from build123d import *

# Parameters (mm, degrees)
SKETCH3_R          = 3.175
CUT_EXTRUDE1_DEPTH = 0.91186
CIRPATTERN1_COUNT  = 8


with BuildPart() as part:
    # Sketch1 → Revolve1 (revolve)
    with BuildSketch(Plane.XY):
        Polygon((-1101.212903226, 25.4), (-1060.572903226, 76.2), (-1040.252903226, 76.2), (-1039.341043226, 76.2), (-1039.341043226, 89.81186), (-1040.252903226, 89.81186), (-1040.252903226, 77.11186), (-1061.011165799, 77.11186), (-1101.924946258, 25.969634426), align=None)
    revolve(axis=Axis((0, 0, 0), (-1, 0, 0)))

    # Sketch3 → Cut-Extrude1 (cut)
    with BuildSketch(Plane.ZY.offset(1040.252903226)):
        with Locations((0, 85.09)):
            Circle(SKETCH3_R)
    cut_extrude1 = extrude(amount=-CUT_EXTRUDE1_DEPTH, mode=Mode.SUBTRACT)

    # CirPattern1: Cut-Extrude1 ×8 about axis
    cirpattern1_axis = Axis((0, 0, 0), (1, 0, 0))
    for i in range(1, CIRPATTERN1_COUNT):
        add(cut_extrude1.rotate(cirpattern1_axis, i * 360 / CIRPATTERN1_COUNT), mode=Mode.SUBTRACT)


solid = part.part
Check sheet for the modelled part. Datum: model origin and axes. Units: mm. A direction names the side the tool comes from. Round coordinates to 2 decimals unless told otherwise and drop trailing zeros. Order: outer loops, then holes, each group sorted by start corner. A loop starts at its lowest first (then second) coordinate and runs counter-clockwise, first axis right, second up. Notation, with made-up numbers: M 38,-10 L 82,-10 A26 ccw 82,20 Z; hole C 16.25,16 d5. An arc over 180 degrees is marked long. One line per item, written item: value. Start each with the question number.
1. Access from +Z, -Z, +X, -X, +Y, -Y to the whole of each face (thin tool, end or side, straight path). Record for faces 4 (the cylindrical face through (-1049.808, -60.47, 46.367)), 5 (the cylindrical face through (-1039.8, 60.03, -63.34)), 6 (the flat face through (-1040.253, 0, 79)).
2. Section check D-D on x = -1051. Enter the section's corners in (y, z), and give its area (3 significant figures).
3. Section check A-A on z = 0. Enter the section's corners in (x, y) (3 decimals), and give its area (3 significant figures).
4. Scan lines: line 1 along Z through (x, y) = (-1039.7, 0) (3 decimals); line 2 along Y through (x, z) = (-1045, 0); line 3 along Z through (x, y) = (-1063, 34.5). Record each from-to range of solid material in increasing order.
5. Release check for a two-part mould opening along Y. For faces 1 (the cylindrical face through (-1039.8, -88.24, 0.41)), 2 (the cylindrical face through (-1050.777, -10.038, -76.456)), 3 (the flat face through (-1039.341, 20, -74)) record: released by +Y, released by -Y, zero draft, split by the parting line, or undercut.
6. Section check C-C on y = -85.09. Enter the section's corners in (x, z) (3 decimals), and give its area (3 significant figures).
7. Gauge pin test, flat ends, axial feed: P1, Ø7.5, axis at y = 85.09, z = 0, coming from the +X side; P2, Ø1.5, axis at x = -1087.5, z = -28, coming from the +Y side; P3, Ø4, axis at y = 60.17, z = 60.17, coming from the -X side; P4, Ø4, axis at y = -46.5, z = -5, coming from the +X side. Record the tip position at first contact, or that the pin passes through.
Results found:
1. face 4: +X
1. face 5: +X, -X
1. face 6: -X
2. outline: C 0,0 d154.22; hole C 0,0 d152.4
2. area: 439 mm^2
3. outline: M -1101.925,-25.97 L -1061.011,-77.112 L -1040.253,-77.112 L -1040.253,-81.915 L -1039.341,-81.915 L -1039.341,-76.2 L -1060.573,-76.2 L -1101.213,-25.4 Z; M -1101.925,25.97 L -1101.213,25.4 L -1060.573,76.2 L -1039.341,76.2 L -1039.341,81.915 L -1040.253,81.915 L -1040.253,77.112 L -1061.011,77.112 Z; M -1040.253,-89.812 L -1039.341,-89.812 L -1039.341,-88.265 L -1040.253,-88.265 Z; M -1040.253,88.265 L -1039.341,88.265 L -1039.341,89.812 L -1040.253,89.812 Z
3. area: 170 mm^2
4. line 1: -89.812 to -88.265, -81.915 to -76.2, 76.2 to 81.915, 88.265 to 89.812
4. line 2: -77.11 to -76.2, 76.2 to 77.11
4. line 3: -66.17 to -64.52, 64.52 to 66.17
5. face 1: undercut
5. face 2: split by the parting line
5. face 3: zero draft
6. outline: M -1040.253,-28.738 L -1039.341,-28.738 L -1039.341,-3.175 L -1040.253,-3.175 Z; M -1040.253,3.175 L -1039.341,3.175 L -1039.341,28.738 L -1040.253,28.738 Z
6. area: 46.6 mm^2
7. P1: x = -1039.34
7. P2: y = 35.29
7. P3: through
7. P4: x = -1082.52
